Here's the drawing with two shaded views (mm, measured from the low corner). I have some questions. A direction names the side the tool comes from. Round coordinates to 2 decimals unless told otherwise and drop trailing zeros. Order: outer loops, then holes, each group sorted by start corner. A loop starts at its lowest first (then second) coordinate and runs counter-clockwise, first axis right, second up. Notation, with made-up numbers: (-15, 58.25) -> (-9, 58.25) arc R19 ccw to (-9, 93.25) -> close; hole circle Ø8 at (41, 1.25). An arc over 180 degrees is marked (long way). One line per question, with ' | ' between items.
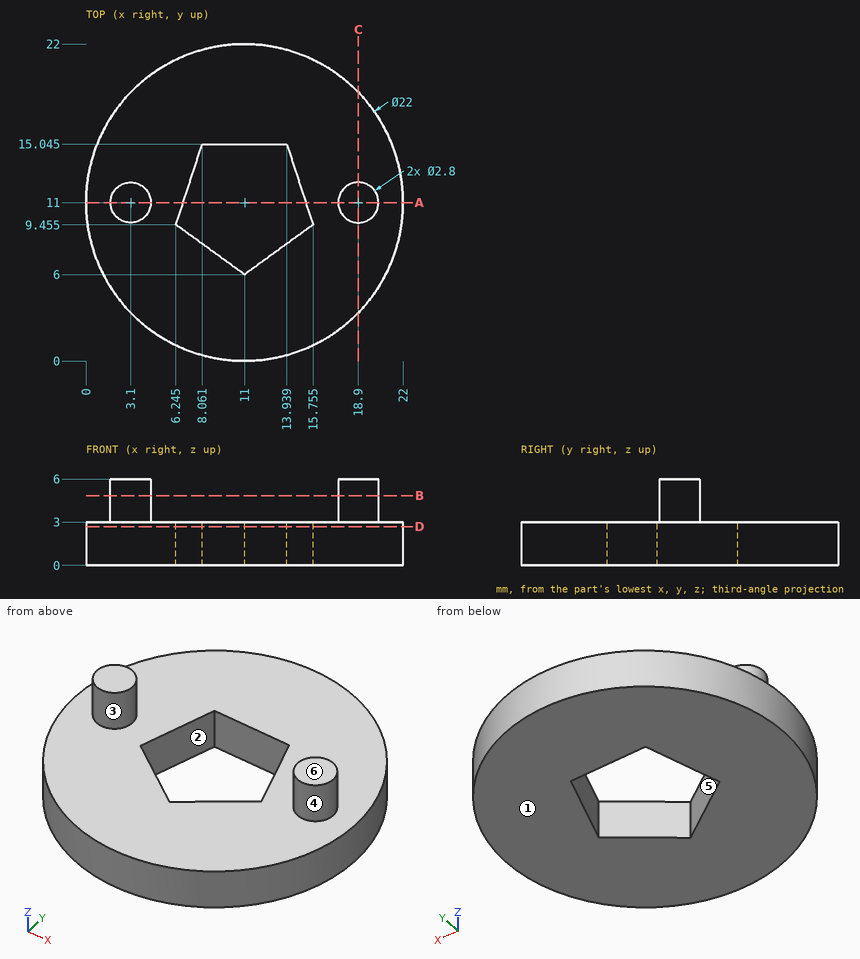
1. I want a section at B-B on z = 4.85. List the corners of the cut face in (x, y) for me.
From the geometry:
outline: circle Ø2.8 at (3.1, 11); circle Ø2.8 at (18.9, 11)
2. I want a section at C-C on x = 18.9. List the corners of the cut face in (y, z) for me.
From the geometry:
outline: (3.35, 0) -> (18.65, 0) -> (18.65, 3) -> (12.4, 3) -> (12.4, 6) -> (9.6, 6) -> (9.6, 3) -> (3.35, 3) -> close
3. I need wall thicknesses on probe 1 along Z at (x, y) = (15.5, 1); probe 2 along Y at (x, z) = (8.5, 2.65) (1 decimal); probe 3 along Y at (x, z) = (12.5, 1.25) (1 decimal). Which ranges of each line are inside material? Lowest first, please.
From the geometry:
probe 1: z = 0 to 3 | probe 2: y = 0.3 to 7.8, 15 to 21.7 | probe 3: y = 0.1 to 7.1, 15 to 21.9
4. I want a section at A-A on y = 11. List the corners of the cut face in (x, z) for me.
From the geometry:
outline: (0, 0) -> (6.75, 0) -> (6.75, 3) -> (4.5, 3) -> (4.5, 6) -> (1.7, 6) -> (1.7, 3) -> (0, 3) -> close; (15.25, 0) -> (22, 0) -> (22, 3) -> (20.3, 3) -> (20.3, 6) -> (17.5, 6) -> (17.5, 3) -> (15.25, 3) -> close
5. On a 3-axis mill with a long thin cutter (end or side, diameter ignored), from which of +Z, -Z, +X, -X, +Y, -Y can I reach the whole of each face in a straight line? I mean the marked faces 4, 5 and 6. Say none if no direction works.
From the geometry:
face 4: +Z | face 5: +Z, -Z | face 6: +Z, +X, -X, +Y, -Y
6. I'm going to push flat-ended pins straight in: pin 1 (1 mm diameter, centred on x = 9.5, z = 2, fed in from +Y); pin 2 (2 mm diameter, centred on x = 9, y = 3.5, fed in from +Z); pin 3 (1.5 mm diameter, centred on x = 2.5, z = 2.5, fed in from +Y). Where does each tip first touch, or does it pass through?
From the geometry:
pin 1: stops at y = 21.95 | pin 2: stops at z = 3 | pin 3: stops at y = 18.81
7. I want a section at D-D on z = 2.7. List the corners of the cut face in (x, y) for me (1 decimal), and give its area (3 significant figures).
From the geometry:
outline: circle Ø22 at (11, 11); hole (6.2, 9.5) -> (11, 6) -> (15.8, 9.5) -> (13.9, 15) -> (8.1, 15) -> close | area: 321 mm²
8. If we mould it in two halves opening along Y, with no side actions, what happens to the marked faces 1, 2 and 3? For each: pulls with the +Y half, pulls with the -Y half, needs draft (parallel to the pull), parting line crosses it, or undercut.
From the geometry:
face 1: needs draft | face 2: undercut | face 3: parting line crosses it
